Geometry: see drawing. Coordinates: mm, zero at the bounding-box minimum. A direction names the side the tool comes from. Give positions to 0.01 mm unless a question says otherwise; leave off trailing zeros. Write each loop counter-clockwise with the first axis right and the second up, starting at its lowest first coordinate (ties: lowest second). Pieces come first, ordered by that corner, then holes.
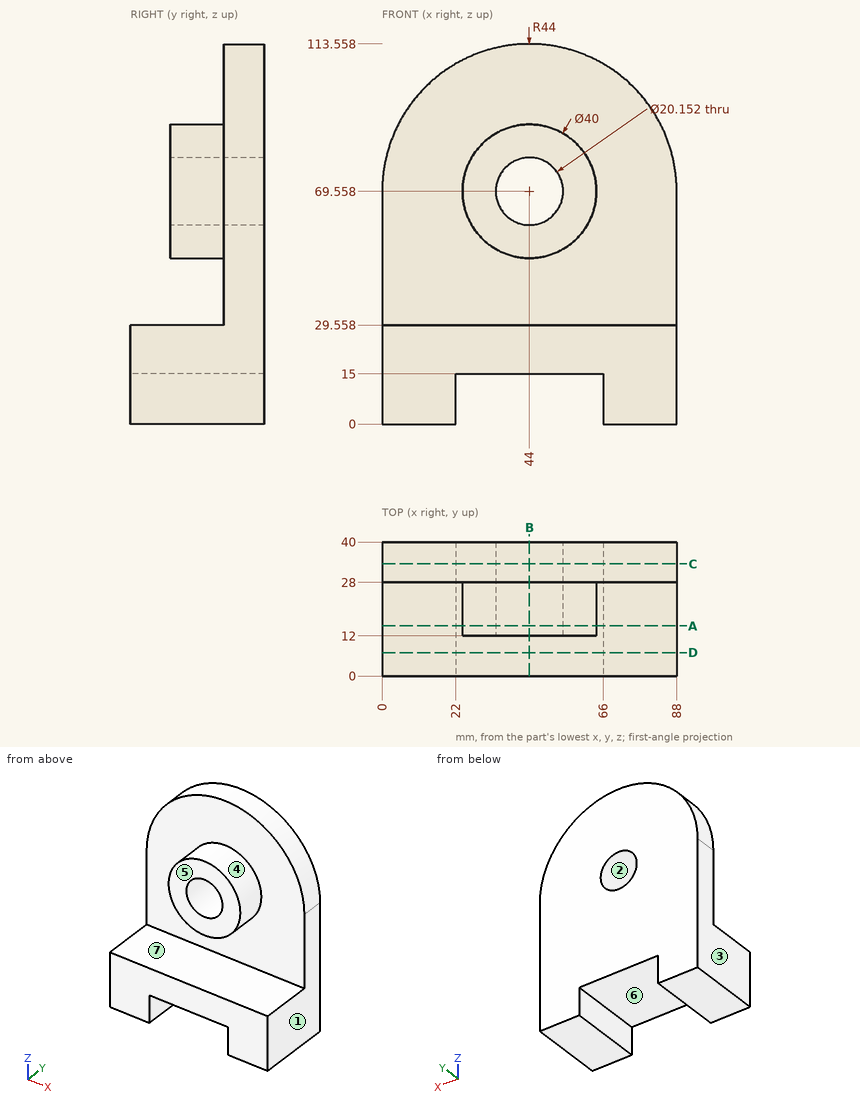
Q1. Section A-A, the plane y = 15. Return the cut outline in (x, z), then the cut area to 3 significant figures.
Q2. Section C-C, the plane y = 33.5. Return the cut outline in (x, z).
Q3. Section B-B, the plane x = 44. Return the cut outline in (y, z), then the cut area to 3 significant figures.
Q4. Pin query (flat end, axial travel): pin 1 (1 mm diameter, centred on x = 49, y = 16, fed in from -Z); pin 2 (12 mm diameter, centred on x = 32, y = 33, fed in from +Z); pin 3 (25 mm diameter, centred on x = 40.5, z = 84.5, fed in from -Y). Return the tip coordinate at first contact, or that it passes through.
Q5. Mould query, pull axis X, two halves, no side actions, for the marked faces 1, 2 and 3. Classes: +X half, -X half, draft (parallel to the pull), parting line (faces both ways), or undercut.
Q6. Access query for the marked faces 4, 5, 6 and 7. Directions: +Z, -Z, +X, -X, +Y, -Y. A direction counts if a zero-diameter tool reaches every point of the face in a straight line with its end or side. Return the directions, or none.
Q7. Section D-D, the plane y = 7. Return the cut outline in (x, z), then the cut area to 3 significant figures.
Q8. Material intervals for line 1 along Z through (x, y) = (44, 22); line 2 along X through (y, z) = (23.5, 12); line 3 along Z through (x, y) = (44, 32), sorted ascending.
Solutions:
1. outline: (0, 0) - (22, 0) - (22, 15) - (66, 15) - (66, 0) - (88, 0) - (88, 29.56) - (0, 29.56) - close; circle Ø40 at (44, 69.56); hole circle Ø20.15 at (44, 69.56)
1. area: 2,880 mm2
2. outline: (0, 0) - (22, 0) - (22, 15) - (66, 15) - (66, 0) - (88, 0) - (88, 69.56) arc R44 ccw to (0, 69.56) - close; hole circle Ø20.15 at (44, 69.56)
3. outline: (0, 15) - (40, 15) - (40, 59.48) - (12, 59.48) - (12, 49.56) - (28, 49.56) - (28, 29.56) - (0, 29.56) - close; (12, 79.63) - (40, 79.63) - (40, 113.56) - (28, 113.56) - (28, 89.56) - (12, 89.56) - close
3. area: 1,670 mm2
4. pin 1: stops at z = 15
4. pin 2: stops at z = 113.15
4. pin 3: stops at y = 12
5. face 1: +X half
5. face 2: undercut
5. face 3: -X half
6. face 4: -Y
6. face 5: +Z, +X, -X, -Y
6. face 6: -Z, +Y, -Y
6. face 7: +X, -X, -Y
7. outline: (0, 0) - (22, 0) - (22, 15) - (66, 15) - (66, 0) - (88, 0) - (88, 29.56) - (0, 29.56) - close
7. area: 1,940 mm2
8. line 1: z = 15 to 29.56, 49.56 to 59.48, 79.63 to 89.56
8. line 2: x = 0 to 22, 66 to 88
8. line 3: z = 15 to 59.48, 79.63 to 113.56
